The listing builds one solid part. Answer for the finished solid, in the listing's coordinates (mm). Face numbers are marked on the shaded views. A direction names the side the tool comes from. Round coordinates to 2 decimals unless told otherwise and drop trailing zeros. Order: outer loops, then holes, each group sorted by start corner. A loop starts at its lowest first (then second) coordinate and runs counter-clockwise, first axis right, second up. Notation, with made-up numbers: M 45.25,-11 L 61.25,-11 A18 ccw 61.25,22 Z; hole C 7,87 d10. An arc over 180 degrees is marked long. Put each result on its own line as item: value. Start each with the question number.
1. The part is cut by section D-D (z = 21.5). Give the vertices of the cut face in (x, y).
2. Each of these flat-tipped pins is pushed along its axis until it touches: pin 1 Ø3 at (x, y) = (20, -17.5) entering from -Z; pin 2 Ø10 at (x, y) = (-22.5, -30.5) entering from +Z. Where does it stop, or does it pass through?
3. Which of the six approach directions +Z, -Z, +X, -X, +Y, -Y give full straight-line access (tool end or side, diameter ignored) to the marked faces 4 and 5?
4. The part is cut by section B-B (z = 40). Give the vertices of the cut face in (x, y), then the cut area to 3 significant figures.
5. The part is cut by section A-A (y = 0). Give the vertices of the cut face in (x, z), then the cut area to 4 significant figures.
6. The mould has two halves that part along Y. Classify the marked faces 1, 2 and 3: +Y half, -Y half, draft (parallel to the pull), parting line (faces both ways), or undercut.
7. The part is cut by section C-C (x = -3.5). Give the vertices of the cut face in (y, z), then the cut area to 4 significant figures.
8. Consider line 1 (Y direction, x = 34, z = 29.5); line 2 (Z direction, x = -6, y = 18). Determine where each line is inside the solid, lowest interval first.
from build123d import *

# Parameters (mm, degrees)
F0_W     = 100
F0_H     = 100
F2_DEPTH = 50
F3_DEPTH = 50
F4_T     = -2.5
F8_DEPTH = 100.001


# Not quite as in the source:
# - a feature names something its author has since deleted; it is built from what else it names


with BuildPart() as f2:
    # F0 (on Front) → F2 (new body)
    with BuildSketch(Plane.XZ):
        with Locations((0, 50)):
            Rectangle(F0_W, F0_H)
    extrude(amount=F2_DEPTH)

    # F3 (add): a face of the model
    f3_faces = [f2.faces().sort_by_distance(p)[0] for p in [
        (0, 0, 50),
    ]]
    extrude(f3_faces, amount=F3_DEPTH)

    # F4
    f4_openings = [f2.faces().sort_by_distance(p)[0] for p in [
        (0, 0, 100),
    ]]
    offset(amount=F4_T, openings=f4_openings)

    # F7 (on offset) → F8 (cut, through all)
    with BuildSketch(Plane.YZ.offset(50)):
        Polygon((25, 75), (-25, 75), (-25, 25), (0, 25), (25, 25), align=None)
    extrude(amount=-F8_DEPTH, mode=Mode.SUBTRACT)


solid = f2.part
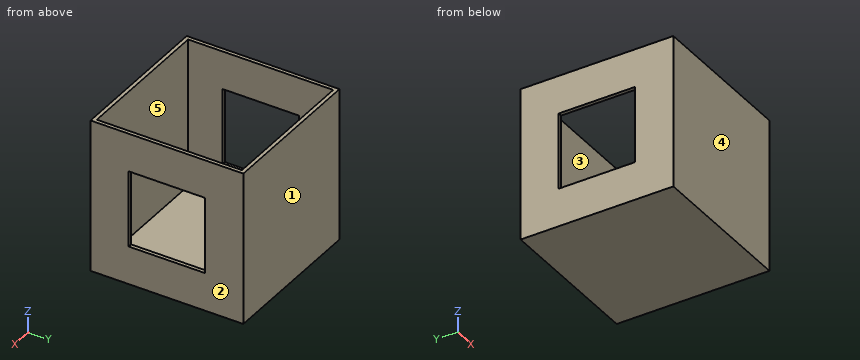
Resolved:
1. outline: M -50,-50 L 50,-50 L 50,50 L -50,50 Z; hole M -47.5,-47.5 L 47.5,-47.5 L 47.5,47.5 L -47.5,47.5 Z
2. pin 1: z = 0
2. pin 2: z = 2.5
3. face 4: +Z, -Z, +X, -X, -Y
3. face 5: +Z
4. outline: M -50,-50 L 50,-50 L 50,-25 L 47.5,-25 L 47.5,-47.5 L -47.5,-47.5 L -47.5,-25 L -50,-25 Z; M -50,25 L -47.5,25 L -47.5,47.5 L 47.5,47.5 L 47.5,25 L 50,25 L 50,50 L -50,50 Z
4. area: 725 mm2
5. outline: M -50,0 L 50,0 L 50,25 L 47.5,25 L 47.5,2.5 L -47.5,2.5 L -47.5,25 L -50,25 Z; M -50,75 L -47.5,75 L -47.5,100 L -50,100 Z; M 47.5,75 L 50,75 L 50,100 L 47.5,100 Z
5. area: 487.5 mm2
6. face 1: +Y half
6. face 2: draft
6. face 3: undercut
7. outline: M -50,0 L 50,0 L 50,100 L 47.5,100 L 47.5,2.5 L -47.5,2.5 L -47.5,100 L -50,100 Z
7. area: 737.5 mm2
8. line 1: -50 to -47.5, 47.5 to 50
8. line 2: 0 to 2.5
